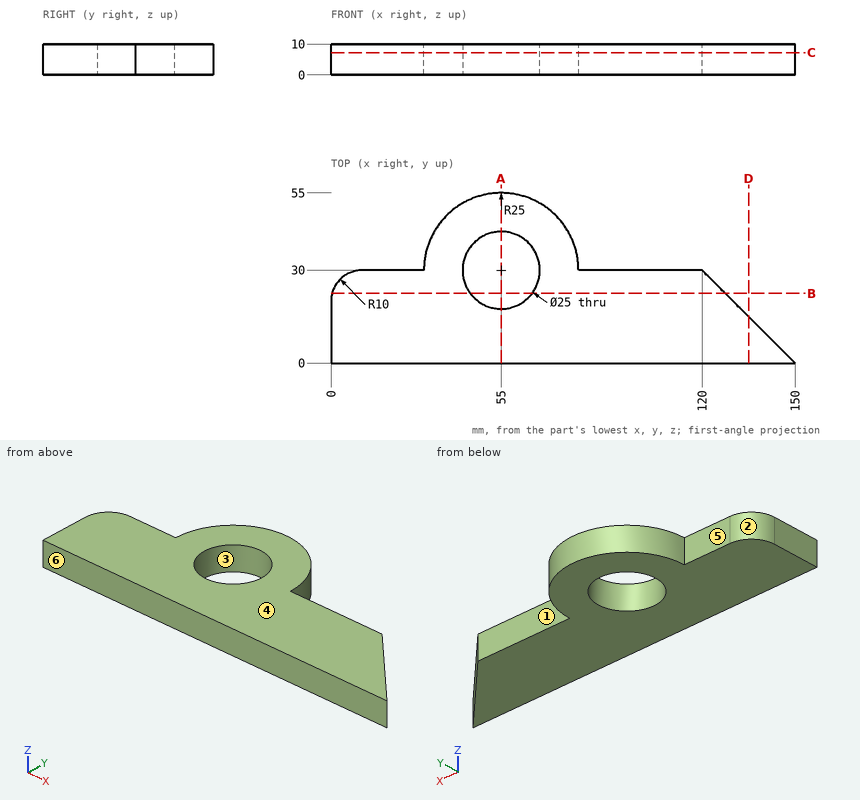
Source: three-view drawing plus pictorial views. Frame: mm from the lowest corner of the part. A direction names the side the tool comes from. Give positions to 0.01 mm unless a question says otherwise; leave off trailing zeros. Loops run counter-clockwise (first coordinate to the right, second up) from the corner with the lowest first, then second, coordinate; pieces in that order, holes last. Notation, with made-up numbers: (-16.5, 49) -> (16.5, 49) arc R13 ccw to (16.5, 62) -> close; hole circle Ø9 at (-24.5, 6.5). An arc over 180 degrees is marked (long way). Use a Markdown table: item, result. Add a question column.
(1) Access query for the marked faces 1 and 2. Directions: +Z, -Z, +X, -X, +Y, -Y. A direction counts if a zero-diameter tool reaches every point of the face in a straight line with its end or side. Return the directions, or none.
(2) Section query C-C (z = 7.25). Output: boundary loops of the cut face in (x, y).
(3) Section query B-B (y = 22.5). Output: boundary loops of the cut face in (x, z), then the cut area to 3 significant figures.
(4) Section query A-A (x = 55). Output: boundary loops of the cut face in (y, z), then the cut area to 3 significant figures.
(5) First-contact query: pin 1 Ø6 at (x, z) = (116, 4.5) entering from +Y; pin 2 Ø2 at (y, z) = (45, 3.5) entering from -X; pin 3 Ø1.5 at (y, z) = (35, 1.5) entering from -X. Flat tips, straight axial feed; report the tip coordinate or a pass-through.
(6) Pull-direction query (Y, two-part tool) for the marked faces 3, 4, 5 and 6; classes: +Y half, -Y half, draft (parallel to the pull), parting line (faces both ways), or undercut.
(7) Ray query, line 1 (Y direction, x = 55, z = 7.5); line 2 (Y direction, x = 82.5, z = 1.25); line 3 (Y direction, x = 59, z = 6.25). Return the intervals inside material, ascending.
(8) Section query D-D (x = 135). Output: boundary loops of the cut face in (y, z), then the cut area to 3 significant figures.
Checked values:
| question | item | result |
|---|---|---|
| 1 | face 1 | +Z, -Z, +X, +Y |
| 1 | face 2 | +Z, -Z, -X, +Y |
| 2 | outline | (0, 0) -> (150, 0) -> (120, 30) -> (80, 30) arc R25 ccw to (30, 30) -> (10, 30) arc R10 ccw to (0, 20) -> close; hole circle Ø25 at (55, 30) |
| 3 | outline | (0.32, 0) -> (45, 0) -> (45, 10) -> (0.32, 10) -> close; (65, 0) -> (127.5, 0) -> (127.5, 10) -> (65, 10) -> close |
| 3 | area | 1,070 mm^2 |
| 4 | outline | (0, 0) -> (17.5, 0) -> (17.5, 10) -> (0, 10) -> close; (42.5, 0) -> (55, 0) -> (55, 10) -> (42.5, 10) -> close |
| 4 | area | 300 mm^2 |
| 5 | pin 1 | y = 30 |
| 5 | pin 2 | x = 34.29 |
| 5 | pin 3 | x = 30.36 |
| 6 | face 3 | undercut |
| 6 | face 4 | draft |
| 6 | face 5 | +Y half |
| 6 | face 6 | -Y half |
| 7 | line 1 | 0 to 17.5, 42.5 to 55 |
| 7 | line 2 | 0 to 30 |
| 7 | line 3 | 0 to 18.16, 41.84 to 54.68 |
| 8 | outline | (0, 0) -> (15, 0) -> (15, 10) -> (0, 10) -> close |
| 8 | area | 150 mm^2 |
